For this review, take the finished solid that the model builds, in its own axes (mm). A direction names the side the tool comes from. Round coordinates to 2 decimals unless told otherwise and drop trailing zeros. Write each loop counter-clockwise with the first axis right and the second up, starting at its lowest first coordinate (ties: lowest second). Pieces come first, ordered by that corner, then holes. Notation, with made-up numbers: M 35,43 L 81,43 A21 ccw 81,57 Z; hole C 75.5,9 d11. An arc over 180 degrees is marked long. One line per question, with ' | ' between items.
```python
from build123d import *

# Parameters (mm, degrees)
CHAMFER_2_R = 0.2
HEX_2_DEPTH = 1.56


with BuildPart() as part:
    # Эскиз1 → Body (revolve)
    with BuildSketch(Plane.XY):
        with BuildLine():
            Line((0, 2.375), (0, 0))
            Line((0, 0), (10.75, 0))
            Line((10.75, 0), (10.75, 2.055))
            Line((10.75, 2.055), (10.305, 2.5))
            Line((10.305, 2.5), (2.75, 2.5))
            Line((2.75, 2.5), (2.75, 4.75))
            Line((2.75, 4.75), (2.370164642, 4.75))
            ThreePointArc((2.370164642, 4.75), (0.992749859, 3.754440885), (0, 2.375))
        make_face()
    revolve(axis=Axis((-3.643489966, 0, 0), (-1, 0, 0)))

    # Chamfer 2
    chamfer_2_edges = [part.edges().sort_by_distance(p)[0] for p in [
        (2.75, -2.5, 0),
    ]]
    fillet(chamfer_2_edges, radius=CHAMFER_2_R)

    # Эскиз2 → Hole (revolve, cut)
    with BuildSketch(Plane.XY):
        Polygon((0, 0), (0, 1.5), (1.56, 1.5), (2.426025404, 0), align=None)
    revolve(axis=Axis((2.426025404, 0, 0), (-1, 0, 0)), mode=Mode.SUBTRACT)

    # Эскиз3 → Hex 2 (cut)
    with BuildSketch(Plane.ZY):
        Polygon((-1.5, -0.866025404), (0, -1.732050808), (1.5, -0.866025404), (1.5, 0.866025404), (0, 1.732050808), (-1.5, 0.866025404), align=None)
    extrude(amount=-HEX_2_DEPTH, mode=Mode.SUBTRACT)


solid = part.part
```
Item 1: Insertion check: pin 1 Ø1 at (x, y) = (7, 0) entering from -Z; pin 2 Ø2 at (y, z) = (1, 3) entering from +X; pin 3 Ø1.7 at (x, y) = (0.5, 0) entering from -Z. Each pin has a flat end and moves straight along its axis. Give the tip position at first contact, or say it passes through.
Results:
pin 1: z = -2.5 | pin 2: x = 10.64 | pin 3: z = -4.08
Item 2: Mouldability with a two-part tool opening along Z and no side actions: class faces 1 (the face through (0.769, -1.293, -0.76)), 2 (the face through (6.58, -0.54, 2.44)), 3 (the face through (0, 0, 2)) as +Z half, -Z half, draft (parallel to the pull), parting line (faces both ways), or undercut.
Results:
face 1: undercut | face 2: parting line | face 3: draft
Item 3: Machinability: for faces 4 (the face through (0.769, 1.293, 0.76)), 5 (the face through (2.75, -2.04, 2.04)), 6 (the face through (2.557, 2.192, 4.214)), which of the approach directions +Z, -Z, +X, -X, +Y, -Y give a long, thin tool a straight path to every point of the face, cutting with its end or side? Answer none if there is none.
Results:
face 4: -X | face 5: +X | face 6: +X, -X
Item 4: Take a section at C-C (x = 3.75). Write out the cut boundary in (y, z).
Results:
outline: C 0,0 d5
Item 5: To check wall thickness, follow line 1 along Y through (x, z) = (6, 0); line 2 along Z through (x, y) = (2.5, 2.75); line 3 along X through (y, z) = (2.25, -0.25). State the ranges of each line that lie inside material, in increasing order. Write a range as from..to.
Results:
line 1: -2.5..2.5 | line 2: -3.87..3.87 | line 3: 0..10.54
Item 6: Take a section at A-A (y = -3). Write out the cut boundary in (x, z), then the cut area to 3 significant figures.
Results:
outline: M 2.37,-3.68 L 2.75,-3.68 L 2.75,3.68 L 2.37,3.68 A4.39 ccw Z | area: 13.2 mm2
Item 7: Take a section at B-B (z = -3.75). Write out the cut boundary in (x, y).
Results:
outline: M 2.37,-2.92 L 2.75,-2.92 L 2.75,2.92 L 2.37,2.92 A3.77 ccw Z
